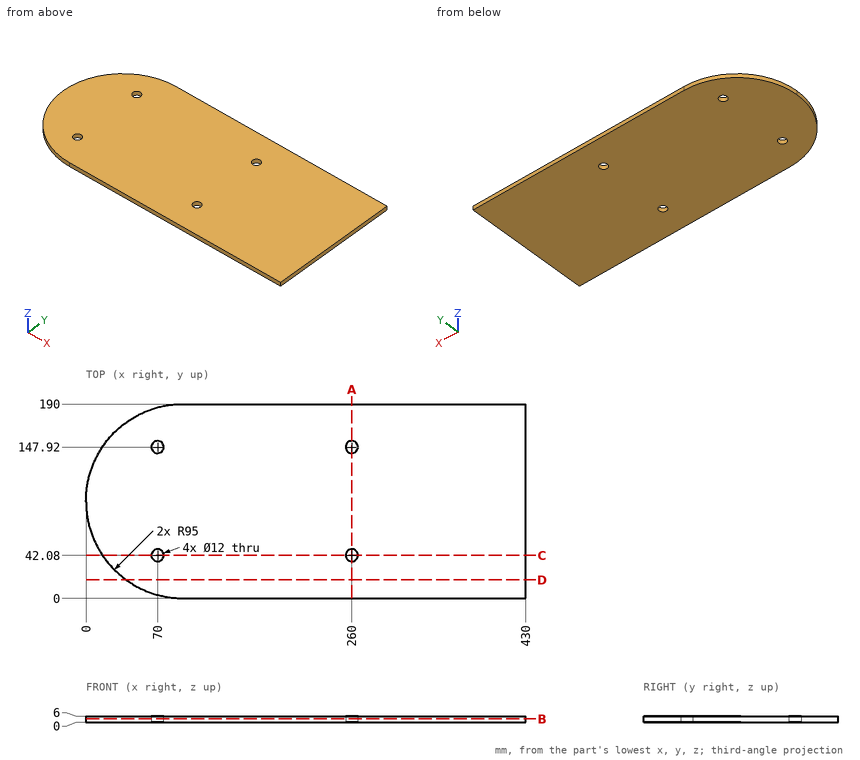
Input: dimensioned drawing with shaded views. Units: mm. Origin: part minimum x, y, z. Coordinates: 2 decimals unless noted, no trailing zeros. Loops run counter-clockwise (first coordinate to the right, second up) from the corner with the lowest first, then second, coordinate; pieces in that order, holes last. Notation, with made-up numbers: M 8.25,16.25 L 34.25,16.25 A12 ccw 34.25,24.25 Z; hole C 57.25,44 d9. An arc over 180 degrees is marked long. Use a Markdown table: item, result. Add a question column.
Q1. First-contact query: pin 1 (7 mm diameter, centred on x = 260, y = 42.08, fed in from -Z); pin 2 (4 mm diameter, centred on x = 294.5, y = 101.5, fed in from -Z); pin 3 (1.5 mm diameter, centred on y = 84.5, z = 3.5, fed in from -X). Flat tips, straight axial feed; report the tip coordinate or a pass-through.
Q2. Section query B-B, the plane z = 3.5. State how many separate pieces and enclosed holes the cut face has, and give its area (3 significant figures).
Q3. Section query D-D, the plane y = 18. Return loops of the section in (x, z), and give its area (3 significant figures).
Q4. Section query C-C, the plane y = 42.08. Return loops of the section in (x, z), and give its area (3 significant figures).
Q5. Material intervals for L1, parallel to Y at x = 260, z = 2.1; L2, parallel to Y at x = 70, z = 2.9; L3, parallel to X at y = 94.5, z = 3.55, sorted ascending.
Q6. Section query A-A, the plane x = 260. Return loops of the section in (y, z).
Result:
| question | item | result |
|---|---|---|
| 1 | pin 1 | passes through |
| 1 | pin 2 | stops at z = 0 |
| 1 | pin 3 | stops at x = 0.5 |
| 2 | separate pieces | 1 |
| 2 | enclosed holes | 4 |
| 2 | area | 77,400 mm2 |
| 3 | outline | M 39.36,0 L 430,0 L 430,6 L 39.36,6 Z |
| 3 | area | 2,340 mm2 |
| 4 | outline | M 16.1,0 L 64,0 L 64,6 L 16.1,6 Z; M 76,0 L 254,0 L 254,6 L 76,6 Z; M 266,0 L 430,0 L 430,6 L 266,6 Z |
| 4 | area | 2,340 mm2 |
| 5 | L1 | y = 0 to 36.08, 48.08 to 141.92, 153.92 to 190 |
| 5 | L2 | y = 3.35 to 36.08, 48.08 to 141.92, 153.92 to 186.65 |
| 5 | L3 | x = 0 to 430 |
| 6 | outline | M 0,0 L 36.08,0 L 36.08,6 L 0,6 Z; M 48.08,0 L 141.92,0 L 141.92,6 L 48.08,6 Z; M 153.92,0 L 190,0 L 190,6 L 153.92,6 Z |
